Design review of the part built by this model. Coordinates are the model's own, in mm. Face numbers are marked on the shaded views. A direction names the side the tool comes from. Round coordinates to 2 decimals unless told otherwise and drop trailing zeros. Loops run counter-clockwise (first coordinate to the right, second up) from the corner with the lowest first, then second, coordinate; pieces in that order, holes last. Notation, with made-up numbers: M 84.25,-18 L 123.25,-18 A20 cw 123.25,20 Z; hole C -7.75,34.25 d2. An arc over 180 degrees is marked long. One line per item, written item: value. Start each with the question number.
Item 1: Mouldability with a two-part tool opening along X and no side actions: class the marked faces 1, 2, 3 and 4 as released by +X, released by -X, zero draft, split by the parting line, or undercut.
Item 2: We need section C-C (x = -9). Write out the cut boundary in (y, z).
Item 3: We need section D-D (y = -15). Write out the cut boundary in (x, z), then the cut area to 3 significant figures.
Item 4: Clearance check with flat-ended pins moving along their axes: pin 1 (2 mm diameter, centred on y = 8.5, z = 8.5, fed in from -X); pin 2 (5 mm diameter, centred on x = -2.5, z = 10, fed in from +Y); pin 3 (9.5 mm diameter, centred on x = -6, z = 14.5, fed in from -Y). State where each tip first meets the part, or that it passes through.
Item 5: For the marked faces 5, 6 and 7, list the 3-axis set-ups (+Z, -Z, +X, -X, +Y, -Y) from which the entire face can be reached by the end or side of a thin tool; tool diameter is ignored.
Item 6: For line 1 along X through (y, z) = (-5.5, 9.75); line 2 along X through (y, z) = (-17, 2); line 3 along Y through (x, z) = (-3, 8), list the stretches that pass through material, from the lowest coordinate up.
Item 7: We need section B-B (y = -22.5). Write out the cut boundary in (x, z), then the cut area to 3 significant figures.
Item 8: We need section A-A (z = 4.75). Write out the cut boundary in (x, y).
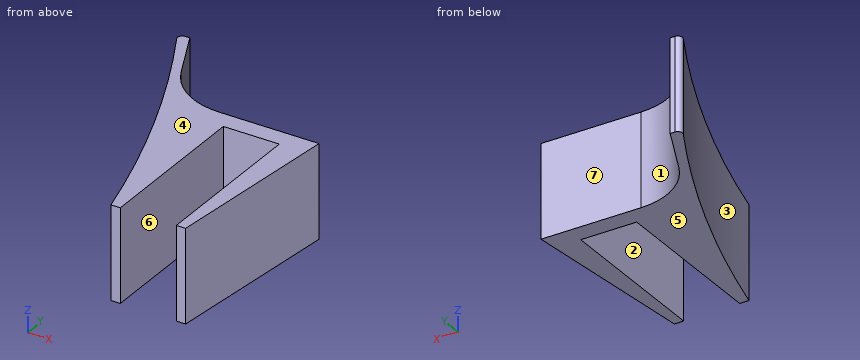
from build123d import *

# Parameters (mm, degrees)
PAD_DEPTH = 20


with BuildPart() as part:
    # Sketch → Pad (new body)
    with BuildSketch(Plane.XY):
        with BuildLine():
            Line((0, 0), (0, -35))
            Line((0, -35), (2, -35))
            Line((2, -35), (6, 4))
            Line((6, 4), (-15.443946, 4))
            ThreePointArc((-29.038563, 12.660726), (-23.50344, 6.349128), (-15.443946, 4))
            Line((-29.038563, 12.660726), (-34.326153, 24))
            Line((-34.326153, 24), (-35.326153, 24))
            ThreePointArc((-35.326153, 24), (-36.184185, 23.513597), (-36.207518, 22.527564))
            ThreePointArc((-14, -35), (-23.323239, -5.548879), (-36.207518, 22.527564))
            Line((-14, -35), (-12, -35))
            Line((-12, -35), (-12, 0))
            Line((-12, 0), (0, 0))
        make_face()
    extrude(amount=PAD_DEPTH)


solid = part.part
A:
1. face 1: released by +X
1. face 2: undercut
1. face 3: released by -X
1. face 4: zero draft
2. outline: M 0,0 L 4,0 L 4,20 L 0,20 Z
3. outline: M -19.89,0 L -12,0 L -12,20 L -19.89,20 Z; M 0,0 L 4.05,0 L 4.05,20 L 0,20 Z
3. area: 239 mm2
4. pin 1: x = -29.71
4. pin 2: y = 4
4. pin 3: y = 0
5. face 5: -Z, +X, -X, +Y, -Y
5. face 6: +Z, -Z, -Y
5. face 7: +Z, -Z, +X, +Y
6. line 1: -23.34 to -12, 0 to 5.03
6. line 2: -19.22 to -12, 0 to 3.85
6. line 3: 0 to 4
7. outline: M -17.47,0 L -12,0 L -12,20 L -17.47,20 Z; M 0,0 L 3.28,0 L 3.28,20 L 0,20 Z
7. area: 175 mm2
8. outline: M -36.21,22.53 A250 cw -14,-35 L -12,-35 L -12,0 L 0,0 L 0,-35 L 2,-35 L 6,4 L -15.44,4 A15 cw -29.04,12.66 L -34.33,24 L -35.33,24 A1 ccw Z
